Check sheet for the drawn part. Datum: minimum x, y, z corner. Units: mm. A direction names the side the tool comes from. Round coordinates to 2 decimals unless told otherwise and drop trailing zeros. Write each loop counter-clockwise with the first axis right and the second up, starting at its lowest first coordinate (ties: lowest second). Pieces come first, ordered by that corner, then holes. Notation, with made-up numbers: M -26.75,80.25 L -16.75,80.25 A18 cw -16.75,93.25 Z; hole C 26.5,-14.5 d8. An arc over 180 degrees is marked long. Put each result on its own line as item: value.
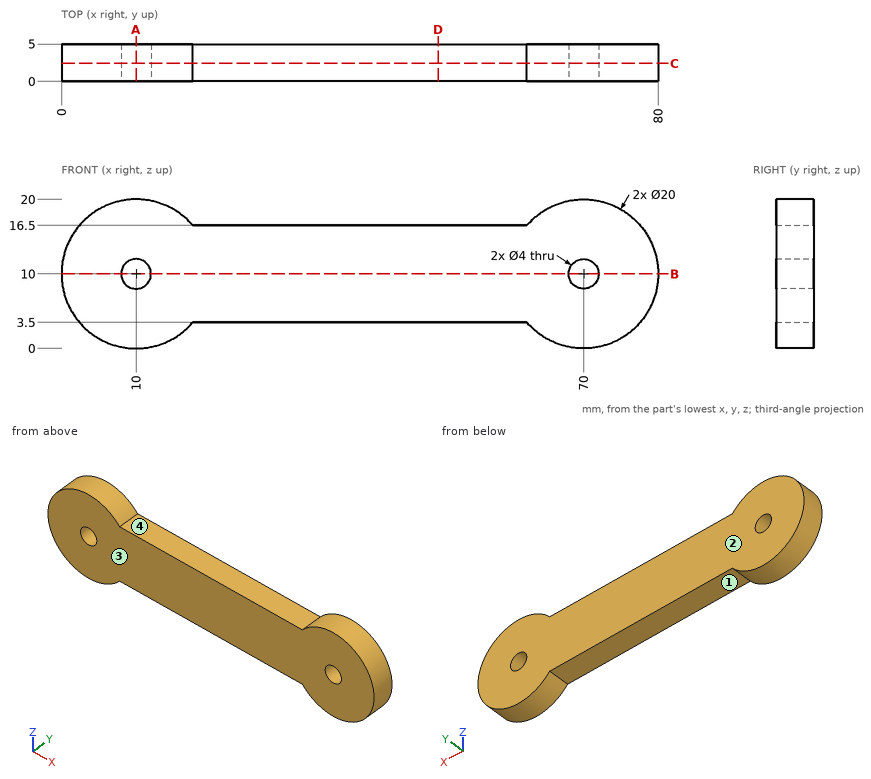
1. Cross-section at B-B (z = 10). Enter the section's corners in (x, y).
Computed values:
outline: M 0,0 L 8,0 L 8,5 L 0,5 Z; M 12,0 L 68,0 L 68,5 L 12,5 Z; M 72,0 L 80,0 L 80,5 L 72,5 Z
2. Scan lines: probe 1 along X at (y, z) = (2.55, 10); probe 2 along Z at (x, y) = (70, 3.65); probe 3 along X at (y, z) = (4.3, 17.75). Record each from-to range of solid material in increasing order.
Computed values:
probe 1: x = 0 to 8, 12 to 68, 72 to 80
probe 2: z = 0 to 8, 12 to 20
probe 3: x = 3.68 to 16.32, 63.68 to 76.32
3. Release check for a two-part mould opening along X. For the marked faces 1 and 2 record: +X half, -X half, draft (parallel to the pull), parting line (faces both ways), or undercut.
Computed values:
face 1: undercut
face 2: draft
4. Cross-section at C-C (y = 2.4). Enter the section's corners in (x, z), then the cut area to 3 significant figures.
Computed values:
outline: M 17.6,3.5 L 62.4,3.5 A10 ccw long 62.4,16.5 L 17.6,16.5 A10 ccw long Z; hole C 10,10 d4; hole C 70,10 d4
area: 1,140 mm2
5. Depth check by flat-ended pin: pin 1 Ø1.5 at (x, y) = (14, 3) entering from -Z; pin 2 Ø3 at (x, z) = (70, 10) entering from -Y. Enter the tip coordinate at first touch or a pass-through.
Computed values:
pin 1: stops at z = 0.54
pin 2: passes through
6. Cross-section at D-D (x = 50.5). Enter the section's corners in (y, z).
Computed values:
outline: M 0,3.5 L 5,3.5 L 5,16.5 L 0,16.5 Z
7. Access from +Z, -Z, +X, -X, +Y, -Y to the whole of each face (thin tool, end or side, straight path). Record for the marked faces 3 and 4.
Computed values:
face 3: +Z, -Z, +X, -X, -Y
face 4: +Z, +Y, -Y
8. Cross-section at A-A (x = 10). Enter the section's corners in (y, z), then the cut area to 3 significant figures.
Computed values:
outline: M 0,0 L 5,0 L 5,8 L 0,8 Z; M 0,12 L 5,12 L 5,20 L 0,20 Z
area: 80.0 mm2
